Part model, mm, in its own coordinate system. A direction names the side the tool comes from. Coordinates: 2 decimals unless noted, no trailing zeros. Order: outer loops, then holes, each group sorted by start corner. A loop starts at its lowest first (then second) coordinate and runs counter-clockwise, first axis right, second up. Notation, with made-up numbers: (70.5, -16.75) - (101.5, -16.75) arc R11 ccw to (101.5, -2.75) - close; hole circle Ø2 at (33, 67.25). An arc over 180 degrees is marked (long way). Use a Markdown table: item, result. Add a question column.
1) Saw through at B-B on z = -105.5. List the corners of the cut face in (x, y), then the cut area to 3 significant figures.
2) Tool access for faces 4 (the face through (0, 3, -42.947)), 5 (the face through (-111.956, 2.535, -52.221)), 6 (the face through (-123, 3, -13.947)), 7 (the face through (120, 3, -7)): list every direction of +Z, -Z, +X, -X, +Y, -Y with a clear straight run to the whole face (end or side of a thin tool).
3) Wall check: L1, parallel to X at y = 1.45, z = -9; L2, parallel to Z at x = 75.5, y = 3.15; L3, parallel to X at y = 0.5, z = -154. Give the ranges that are in metal, low to high. Write a range as [from, to].
4) Two-plate mould, pull along X, no slides. Class faces 1 (the face through (120, 3, -30)), 2 (the face through (-5, 3, -45)), 3 (the face through (-120, 3, -7)): +X half, -X half, draft (parallel to the pull), parting line (faces both ways), or undercut.
5) Saw through at C-C on x = 62.5. List the corners of the cut face in (y, z).
6) Drop flat-ended pins along their axis: P1, Ø1.5, axis at x = 122, y = 2, coming from the +Z side; P2, Ø2.5, axis at y = 3, z = -30, coming from the -X side; P3, Ø2.5, axis at y = 2, z = -8.5, coming from the +X side. Give the stop position or say it passes through.
7) Saw through at A-A on y = 2.35. Count the separate pieces of the cut face and the enclosed holes in it, then the cut area to 3 significant figures.
```python
from build123d import *

# Parameters (mm, degrees)
BOSS_EXTRUDE1_DEPTH = 5
SKETCH2_W           = 5
SKETCH2_H           = 14
SKETCH2_W_2         = 10
SKETCH2_H_2         = 5
CUT_EXTRUDE1_DEPTH  = 210.418973113


with BuildPart() as part:
    # Sketch1 → Boss-Extrude1 (new body)
    with BuildSketch(Plane(origin=(0, 0, 0), x_dir=(1, 0, 0), z_dir=(0, 1, 0))):
        Polygon((-57.5, 167.947331922), (57.5, 167.947331922), (125, 37.947331922), (125, -0.052668078), (-125, -0.052668078), (-125, 37.947331922), align=None)
    extrude(amount=BOSS_EXTRUDE1_DEPTH)

    # Sketch2 → Cut-Extrude1 (cut, through all)
    with BuildSketch(Plane(origin=(0, 5, 0), x_dir=(1, 0, 0), z_dir=(0, 1, 0))):
        Polygon((-77.788864465, 128.872481842), (-103.476511391, 79.39997665), (-99.075067661, 77.027785029), (-73.843707474, 125.621215804), (-73.351788432, 126.56861544), align=None)
        Polygon((-125, 37.947331922), (-125, 23.947331922), (-120, 23.947331922), (-120, 36.728164098), (-103.683242772, 68.152835894), (-108.083917213, 70.526454327), align=None)
        with Locations((-122.5, 6.947331922)):
            Rectangle(SKETCH2_W, SKETCH2_H)
        with Locations((0, 45.447331922)):
            Rectangle(SKETCH2_W_2, SKETCH2_H_2)
        Polygon((-8.411070301, 132.656760174), (-13.226399097, 133.599762064), (-15.148227411, 123.786170675), (-10.332898614, 122.843168786), align=None)
        Polygon((10.332898614, 122.843168786), (15.148227411, 123.786170675), (13.226399097, 133.599762064), (8.411070301, 132.656760174), align=None)
        Polygon((-73.180711758, 137.74744261), (-68.74270223, 135.443091446), (-51.865499988, 167.947331922), (-57.5, 167.947331922), align=None)
        Polygon((73.351788432, 126.56861544), (73.843707474, 125.621215804), (99.075067661, 77.027785029), (103.476511391, 79.39997665), (77.788864465, 128.872481842), align=None)
        Polygon((68.74270223, 135.443091446), (73.180711758, 137.74744261), (57.5, 167.947331922), (51.865499988, 167.947331922), align=None)
        with Locations((122.5, 6.947331922)):
            Rectangle(SKETCH2_W, SKETCH2_H)
        Polygon((125, 23.947331922), (125, 37.947331922), (108.083917213, 70.526454327), (103.683242772, 68.152835894), (120, 36.728164098), (120, 23.947331922), align=None)
    extrude(amount=-CUT_EXTRUDE1_DEPTH, mode=Mode.SUBTRACT)


solid = part.part
```
Results are:
| question | item | result |
|---|---|---|
| 1 | outline | (-84.29, 0) - (84.29, 0) - (84.29, 5) - (-84.29, 5) - close |
| 1 | area | 843 mm2 |
| 2 | face 4 | +Y, -Y |
| 2 | face 5 | -X, +Y, -Y |
| 2 | face 6 | +Z, -X, +Y, -Y |
| 2 | face 7 | +Z, +X, +Y, -Y |
| 3 | L1 | [-120, 120] |
| 3 | L2 | [-133.28, -127.68], [-122.43, 0.05] |
| 3 | L3 | [-59.11, 59.11] |
| 4 | face 1 | +X half |
| 4 | face 2 | undercut |
| 4 | face 3 | -X half |
| 5 | outline | (0, -147.47) - (5, -147.47) - (5, 0.05) - (0, 0.05) - close |
| 6 | P1 | z = -13.95 |
| 6 | P2 | x = -120 |
| 6 | P3 | x = 120 |
| 7 | separate pieces | 1 |
| 7 | enclosed holes | 3 |
| 7 | area | 31,500 mm2 |
